Part model, mm, in its own coordinate system. Round coordinates to 2 decimals unless told otherwise and drop trailing zeros. Order: outer loops, then holes, each group sorted by start corner. A loop starts at its lowest first (then second) coordinate and runs counter-clockwise, first axis right, second up. Notation, with made-up numbers: (-24, 53) -> (4, 53) arc R19 cw to (4, 77) -> close; hole circle Ø8 at (41.5, -16.75). An arc over 180 degrees is marked (long way). Return JSON: item names as keys, results as strings. Group by question number.
Autodesk Inventor part; units mm, degrees
ref_plane "YZ Plane" through (0, 0, 0) normal (1, 0, 0) x (0, 1, 0)
ref_plane "XZ Plane" through (0, 0, 0) normal (0, 1, 0) x (-1, 0, 0)
ref_plane "XY Plane" through (0, 0, 0) normal (0, 0, 1) x (1, 0, 0)
sketch "Sketch1" plane through (0, 0, 0) normal (0, 1, 0) x (-1, 0, 0)
  line L0 (10, -35) -> (-10, -35)
  line L1 (-10, -35) -> (-10, 39.4211)
  line L2 (10, 39.4211) -> (10, -35)
  arc A0 (-10, 39.4211) -> (10, 39.4211) centre (0, 45.1) ccw
  point P0 (0, 0)
  dimension "d2" = 35
  dimension "d3" = 10
  dimension "d36" = 23
  dimension "d37" = 80.1
  dimension "d39" = 74.4211
  dimension "d40" = 20
extrude "Plate1" add sketch "Sketch1" along normal blind 1.5
sketch "Sketch3" plane through (0, 1.5, 0) normal (0, 1, 0) x (1, 0, 0)
  circle A0 centre (0, 25) radius 10
  circle A1 centre (0, -25) radius 10
  line L0 (-10, 35) -> (10, 35)
  line L1 (10, -44) -> (-10, -44)
  line L2 (-10, 35) -> (10, 35)
  line L3 (10, 35) -> (10, 25)
  line L4 (10, 25) -> (-10, 25)
  line L5 (-10, 25) -> (-10, 35)
  line L6 (10, -35) -> (-10, -35)
  line L7 (-10, -35) -> (-10, -25)
  line L8 (-10, -25) -> (10, -25)
  line L9 (10, -25) -> (10, -44)
  point P0 (0, 0)
  point P1 (-10, -39.4211)
  point P2 (10, -25)
  point P3 (0, -35)
  point P4 (-10, -35)
  point P5 (0, 35)
  point P6 (10, 35)
  dimension "d12" = 20
  dimension "d13" = 20
  dimension "d14" = 10
  dimension "d15" = 10
  dimension "d16" = 25
  dimension "d17" = 25
  dimension "d18" = 10
extrude "Extrusion1" cut sketch "Sketch3" against normal blind 10 contours L5 L0 A0 | A0 L0 L3
sketch "Sketch4" plane through (0, 1.5, 0) normal (0, 1, 0) x (1, 0, 0)
  circle A0 centre (-7, 25) radius 0.8
  arc A1 (10, 25) -> (-10, 25) centre (0, 25) ccw
  circle A2 centre (0, 18) radius 0.8
  circle A3 centre (7, 25) radius 0.8
  circle A4 centre (0, 32) radius 0.8
  point P0 (0, 0)
  dimension "d21" = 0
  dimension "d22" = 7
  dimension "d23" = 1.6
  dimension "d26" = 360
hole "Hole2" at (0, 1.5, -32) at (7, 1.5, -25) at (0, 1.5, -18) at (-7, 1.5, -25) direction (0, -1, 0) diameter 2.1 depth 1.5
fillet "Fillet1" radius 1 2 edges at (-10, 0.75, 39.4211) (10, 0.75, 39.4211)
sketch "Sketch5" plane through (0, 1.5, 0) normal (0, 1, 0) x (1, 0, 0)
  arc A0 (10, 25) -> (-10, 25) centre (0, 25) ccw
  point P0 (0, 0)
hole "Hole3" at (0, 1.5, -25) direction (0, -1, 0) diameter 7.2 depth 1.5
sketch "Sketch8" plane through (0, 1.5, 0) normal (0, 1, 0) x (1, 0, 0)
  line L0 (19.8447, -20.3636) -> (-14.9774, -40.4682)
  arc A0 (8.28, -37.1193) -> (-8.28, -37.1193) centre (0, -45.1) ccw
  arc A1 (8.28, -37.1193) -> (10, -36.4253) centre (9, -36.4253) ccw
  line L1 (10, 25) -> (10, -36.4253)
  point P0 (0, 0)
  point P1 (10, -26.0474)
  point P2 (-5.75, -35.1407)
  dimension "d63" = 60
extrude "Extrusion2" cut sketch "Sketch8" against normal blind 1.5
equation "\"d33\" = Thickness"
equation "\"d47\" = Thickness"
equation "\"d4\" = Thickness"
equation "\"BendReliefWidth\" = Thickness"
equation "\"BendReliefDepth\" = 0.5 * Thickness"
equation "\"CornerReliefSize\" = 4 * Thickness"
equation "\"MinimumRemnant\" = 2 * Thickness"
equation "\"TransitionRadius\" = BendRadius"
equation "\"JacobiRadiusSize\" = BendRadius"
equation "\"GapSize\" = Thickness"
properties part number "axis_8_10_connector_frame" material "Aluminum 6061-AHC"
(1) Saw through at D-D, the plane z = 32. List the corners of the cut face in (x, y).
(2) Saw through at C-C, the plane x = 7. List the corners of the cut face in (y, z).
(3) Saw through at B-B, the plane y = 1.05. List the corners of the cut face in (x, z), and give its area (3 significant figures).
(4) Probe L1, parallel to X at y = 1.1, z = -25; L2, parallel to Z at x = 0, y = 1.25; L3, parallel to X at y = 1, z = -18. List the from-to ranges inside material, lowest first. Write a range as [from, to].
(5) Saw through at A-A, the plane z = -18. List the corners of the cut face in (x, y).
(6) Pin check, flat tip, straight feed: P1, Ø1.9, axis at x = 0, z = -32, coming from the -Y side. Stop position of the tip, or through.
(7) Mould opens along X. For faces 1 (the cylindrical face through (0, 1, -35)), 2 (the cylindrical face through (-0.05, 0.74, -19.05)), 3 (the cylindrical face through (-7.102, 0.74, 36.055)) say: pulls with the +X half, pulls with the -X half, needs draft (parallel to the pull), parting line crosses it, or undercut.
Results are:
{
 "1": {"outline": "(-10, 0) -> (-0.31, 0) -> (-0.31, 1.5) -> (-10, 1.5) -> close"},
 "2": {"outline": "(0, -32.14) -> (1.5, -32.14) -> (1.5, -26.05) -> (0, -26.05) -> close; (0, -23.95) -> (1.5, -23.95) -> (1.5, 27.78) -> (0, 27.78) -> close"},
 "3": {"outline": "(-10, -25) arc R10 ccw to (10, -25) -> (10, 26.05) -> (-5.75, 35.14) arc R11.5 cw to (-8.28, 37.12) arc R1 ccw to (-10, 36.43) -> close; hole circle Ø2.1 at (-7, -25); hole circle Ø7.2 at (0, -25); hole circle Ø2.1 at (0, -32); hole circle Ø2.1 at (0, -18); hole circle Ø2.1 at (7, -25)", "area": "1,240 mm^2"},
 "4": {"L1": "x = [-10, -8.05], [-5.95, -3.6], [3.6, 5.95], [8.05, 10]", "L2": "z = [-35, -33.05], [-30.95, -28.6], [-21.4, -19.05], [-16.95, 31.82]", "L3": "x = [-10, -1.05], [1.05, 10]"},
 "5": {"outline": "(-10, 0) -> (-1.05, 0) -> (-1.05, 1.5) -> (-10, 1.5) -> close; (1.05, 0) -> (10, 0) -> (10, 1.5) -> (1.05, 1.5) -> close"},
 "6": {"P1": "passes through"},
 "7": {"face 1": "parting line crosses it", "face 2": "undercut", "face 3": "pulls with the +X half"}
}
